Autodesk Inventor part; units mm, degrees
ref_plane "YZ Plane" through (0, 0, 0) normal (1, 0, 0) x (0, 1, 0)
ref_plane "XZ Plane" through (0, 0, 0) normal (0, 1, 0) x (-1, 0, 0)
ref_plane "XY Plane" through (0, 0, 0) normal (0, 0, 1) x (1, 0, 0)
sketch "Sketch1" plane through (0, 0, 0) normal (0, 0, 1) x (1, 0, 0)
  line L0 (-38.1, -25.4) -> (38.1, -25.4)
  line L1 (38.1, -25.4) -> (38.1, 25.4)
  line L2 (38.1, 25.4) -> (-38.1, 25.4)
  line L3 (-38.1, 25.4) -> (-38.1, -25.4)
  line L4 (-38.1, -25.4) -> (38.1, 25.4) construction
  line L5 (38.1, -25.4) -> (-38.1, 25.4) construction
  point P0 (0, 0)
  dimension "d0" = 76.2
  dimension "d1" = 50.8
extrude "Extrusion1" add sketch "Sketch1" along normal blind 6.35
sketch "Sketch3" plane through (38.1, -25.4, 0) normal (1, 0, 0) x (0, 0, -1)
  line L0 (0, 0) -> (0, 50.8)
  line L1 (0, 50.8) -> (-6.35, 50.8)
  line L2 (-6.35, 0) -> (-6.35, 50.8)
  line L3 (0, 0) -> (-6.35, 0)
  point P0 (0, 25.4)
extrude "Extrusion3" cut sketch "Sketch3" against normal blind 15.875
sketch "Sketch4" plane through (-38.1, -25.4, 0) normal (-1, 0, 0) x (0, 0, 1)
  line L0 (6.35, 16.7952) -> (0, 16.7952)
  line L1 (0, 16.7952) -> (0, 33.2952)
  line L2 (0, 33.2952) -> (6.35, 33.2952)
  line L3 (6.35, 33.2952) -> (6.35, 16.7952)
  line L4 (6.35, 16.7952) -> (0, 33.2952) construction
  line L5 (0, 16.7952) -> (6.35, 33.2952) construction
  line L6 (6.35, 50.8) -> (6.35, 0)
  line L7 (6.35, 50.8) -> (3.175, 50.8)
  line L8 (0, 50.8) -> (6.35, 50.8)
  line L9 (3.175, 50.8) -> (3.175, 25.0452)
  point P0 (0, 25.4)
  dimension "d9" = 6.35
  dimension "d10" = 16.5
extrude "Extrusion4" add sketch "Sketch4" along normal blind 3.302 contours L0 L1 L2 L3
chamfer "Chamfer1" distance 6.35 angle 45 4 edges at (-38.1, -25.4, 3.175) (-38.1, 25.4, 3.175) (22.225, -25.4, 3.175) (22.225, 25.4, 3.175)
sketch "Sketch6" plane through (0, 0, 6.35) normal (0, 0, 1) x (1, 0, 0)
  line L0 (5.9693, 11.0167) -> (6.0307, -10.9832)
  line L1 (-6.0307, 10.9832) -> (6.0307, 10.9832)
  line L2 (6.0307, 10.9832) -> (6.0307, -10.9832)
  line L3 (6.0307, -10.9832) -> (-6.0307, -10.9832)
  line L4 (-6.0307, -10.9832) -> (-6.0307, 10.9832)
  point P0 (0, 0)
  point P1 (5.9694, 10.9832)
extrude "Extrusion5" cut sketch "Sketch6" against normal up to surface (6.35 mm away) contours L0 L3 L4 L1
sketch "Sketch7" plane through (0, 0, 6.35) normal (0, 0, 1) x (1, 0, 0)
  circle A0 centre (-17.4683, 8.1506) radius 2
  circle A1 centre (-17.4683, -8.8674) radius 2
  line L0 (-8.7307, -16.3858) -> (-26.0507, -16.3858)
  line L1 (-8.7307, -16.3858) -> (-8.7307, 15.669)
  line L2 (-8.7307, 15.669) -> (-26.0507, 15.669)
  line L3 (-26.0507, -16.3858) -> (-26.0507, 15.669)
  circle A2 centre (-17.4683, 8.1506) radius 2
  circle A3 centre (-17.4683, -8.8674) radius 2
  point P0 (0, 0)
  dimension "d21" = 4
  dimension "d22" = 4
extrude "Extrusion6" cut sketch "Sketch7" against normal up to surface (6.35 mm away) contours A0 | A1
sketch "Sketch8" plane through (-41.402, -25.4, 0) normal (-1, 0, 0) x (0, 0, 1)
  line L0 (6.35, 16.7952) -> (6.35, 33.2952)
  line L1 (6.35, 33.2952) -> (0, 33.2952)
  line L2 (0, 33.2952) -> (0, 16.7952)
  line L3 (0, 16.7952) -> (6.35, 16.7952)
  line L4 (6.35, 16.7952) -> (6.35, 33.2952)
  line L5 (6.35, 33.2952) -> (0, 33.2952)
  line L6 (0, 33.2952) -> (0, 16.7952)
  line L7 (0, 16.7952) -> (6.35, 16.7952)
  point P0 (0, 25.4)
extrude "Extrusion7" add sketch "Sketch8" along normal blind 12.7
sketch "Sketch9" plane through (-38.1, -8.6048, 0) normal (0, 0, -1) x (1, 0, 0)
  line L0 (0, 0) -> (0, -16.5)
  line L1 (0, 0) -> (0, -8.25)
  line L2 (0, 0) -> (-16.002, 0)
  circle A0 centre (-4.3815, -8.25) radius 2.25
  circle A1 centre (-13.1445, -8.25) radius 2.25
  line L3 (0, -8.25) -> (-4.3815, -8.25)
  line L4 (-4.3815, -8.25) -> (-13.1445, -8.25)
  point P0 (38.1, -8.6048)
  dimension "d28" = 4.5
  dimension "d31" = 4.5
  dimension "d36" = 4.3815
  dimension "d37" = 8.763
sketch "Sketch10" plane through (-54.102, -25.4, 0) normal (-1, 0, 0) x (0, 0, 1)
  line L0 (6.35, 16.7952) -> (6.35, 33.2952)
  line L1 (6.35, 33.2952) -> (0, 33.2952)
  line L2 (0, 33.2952) -> (0, 16.7952)
  line L3 (0, 16.7952) -> (6.35, 16.7952)
  point P0 (0, 25.4)
extrude "Extrusion8" add sketch "Sketch10" along normal blind 3.1877
extrude "Extrusion9" cut sketch "Sketch9" against normal up to surface (6.35 mm away)
sketch "Sketch11" plane through (0, 0, 6.35) normal (0, 0, 1) x (1, 0, 0)
  line L0 (-6.0307, 10.9832) -> (5.9694, 10.9832)
  line L1 (5.9694, 10.9832) -> (6.0307, -10.9832)
  line L2 (-6.0307, -10.9832) -> (-6.0307, 10.9832)
  line L3 (6.0307, -10.9832) -> (-6.0307, -10.9832)
  line L4 (6.2226, 11.2372) -> (-6.2847, 11.2372)
  line L5 (-6.2847, 11.2372) -> (-6.2847, -11.2372)
  line L6 (-6.2847, -11.2372) -> (6.2854, -11.2372)
  line L7 (6.2854, -11.2372) -> (6.2226, 11.2372)
  line L8 (6.2226, 11.2372) -> (-6.2847, 11.2372)
  line L9 (-6.2847, 11.2372) -> (-6.2847, 11.396)
  line L10 (-6.2847, 11.396) -> (6.2226, 11.396)
  line L11 (6.2226, 11.396) -> (6.2226, 11.2372)
  line L12 (6.2854, -11.2372) -> (-6.2876, -11.2372)
  line L13 (-6.2876, -11.2372) -> (-6.2876, -11.396)
  line L14 (-6.2876, -11.396) -> (6.2854, -11.396)
  line L15 (6.2854, -11.396) -> (6.2854, -11.2372)
  point P0 (0, 0)
  dimension "d38" = 0.254
  dimension "d41" = 0.1588
  dimension "d42" = 12.573
  dimension "d43" = 0.1588
extrude "Extrusion10" cut sketch "Sketch11" against normal up to surface (6.35 mm away) contours L7 L6 L5 L4
sketch "Sketch12" plane through (0, 0, 6.35) normal (0, 0, 1) x (1, 0, 0)
  line L0 (6.2226, 11.2372) -> (-6.2847, 11.2372)
  line L1 (-6.2847, 11.2372) -> (-6.2847, -11.2372)
  line L2 (-6.2847, -11.2372) -> (6.2854, -11.2372)
  line L3 (6.2854, -11.2372) -> (6.2226, 11.2372)
  line L4 (6.2226, 11.2372) -> (-6.2847, 11.2372)
  line L5 (-6.2847, 11.2372) -> (-6.2847, 11.396)
  line L6 (-6.2847, 11.396) -> (6.2226, 11.396)
  line L7 (6.2226, 11.396) -> (6.2226, 11.2372)
  line L8 (6.2854, -11.2372) -> (-6.2876, -11.2372)
  line L9 (-6.2876, -11.2372) -> (-6.2876, -11.396)
  line L10 (-6.2876, -11.396) -> (6.2854, -11.396)
  line L11 (6.2854, -11.396) -> (6.2854, -11.2372)
  point P0 (0, 0)
  point P1 (-6.2847, 11.2372)
  dimension "d44" = 0.1588
  dimension "d45" = 12.573
  dimension "d46" = 0.1588
extrude "Extrusion11" cut sketch "Sketch12" against normal up to surface (6.35 mm away) contours L0 L5 L6 L7 | L11 L10 L9 L8 L2
sketch "Sketch13" plane through (0, 0, 6.35) normal (0, 0, 1) x (1, 0, 0)
  line L0 (-6.2847, 11.396) -> (-3.1097, 11.396)
  line L1 (-6.2847, 11.396) -> (6.2226, 11.396)
  line L2 (-6.2847, 11.396) -> (-3.1097, 11.396) construction
  line L3 (6.2226, 11.396) -> (3.0476, 11.396)
  line L4 (-3.1097, 11.396) -> (3.0476, 11.396)
  line L5 (3.0476, 11.396) -> (3.0476, 12.9835)
  line L6 (3.0476, 12.9835) -> (-3.1097, 12.9835)
  line L7 (-3.1097, 12.9835) -> (-3.1097, 11.396)
  point P0 (0, 0)
  dimension "d49" = 3.175
  dimension "d50" = 0
  dimension "d51" = 3.175
  dimension "d52" = 1.5875
extrude "Extrusion12" cut sketch "Sketch13" against normal up to surface (6.35 mm away)
properties part number "Servo Holder Module"
The model under review builds one solid part; all positions refer to its coordinate system, in mm. A direction names the side the tool comes from. Round coordinates to 2 decimals unless told otherwise and drop trailing zeros. Write each loop counter-clockwise with the first axis right and the second up, starting at its lowest first coordinate (ties: lowest second). Pieces come first, ordered by that corner, then holes.
(1) Machinability: for faces 1 (the flat face through (-38.1, 14, 3)), 2 (the flat face through (0, 12.984, 3)), 3 (the flat face through (-48, -8.605, 3)), which of the approach directions +Z, -Z, +X, -X, +Y, -Y give a long, thin tool a straight path to every point of the face, cutting with its end or side? Answer none if there is none.
(2) We need section A-A on x = 1. Give the boundary of the cut face in (y, z).
(3) We need section C-C on y = 3. Give the boundary of the cut face in (x, z) (3 decimals).
(4) Insertion check: pin 1 (5 mm diameter, centred on x = -42.48, y = -0.35, fed in from +Z); pin 2 (3 mm diameter, centred on x = -43.5, z = 4, fed in from -Y); pin 3 (0.8 mm diameter, centred on y = 12, z = 4.5, fed in from -X). Each pin has a flat end and moves straight along its axis. Give the tip position at first contact, or say it passes through.
(5) We need section B-B on z = 5. Give the number of separate pieces and of enclosed holes in the cut face, and give its area (3 significant figures).
(6) Wall thickness on L1, parallel to Y at x = -17.5, z = 1.75; L2, parallel to X at y = -1, z = 4.75 (3 decimals); L3, parallel to X at y = 5.5, z = 5.5 (3 decimals): over which ranges is each line inside the solid? List them lowest first.
Findings below:
1. face 1: +Z, -Z, -X, +Y
1. face 2: +Z, -Z
1. face 3: +Z, -Z, -X, -Y
2. outline: (-25.4, 0) - (-11.4, 0) - (-11.4, 6.35) - (-25.4, 6.35) - close; (12.98, 0) - (25.4, 0) - (25.4, 6.35) - (12.98, 6.35) - close
3. outline: (-57.29, 0) - (-6.285, 0) - (-6.285, 6.35) - (-57.29, 6.35) - close; (6.246, 0) - (22.225, 0) - (22.225, 6.35) - (6.246, 6.35) - close
4. pin 1: stops at z = 6.35
4. pin 2: stops at y = -8.6
4. pin 3: stops at x = -38.1
5. separate pieces: 1
5. enclosed holes: 5
5. area: 2,950 mm2
6. L1: y = -25.4 to -10.87, -6.87 to 6.15, 10.15 to 25.4
6. L2: x = -57.29 to -53.4, -49.089 to -44.637, -40.326 to -6.285, 6.257 to 22.225
6. L3: x = -57.29 to -6.285, 6.239 to 22.225
